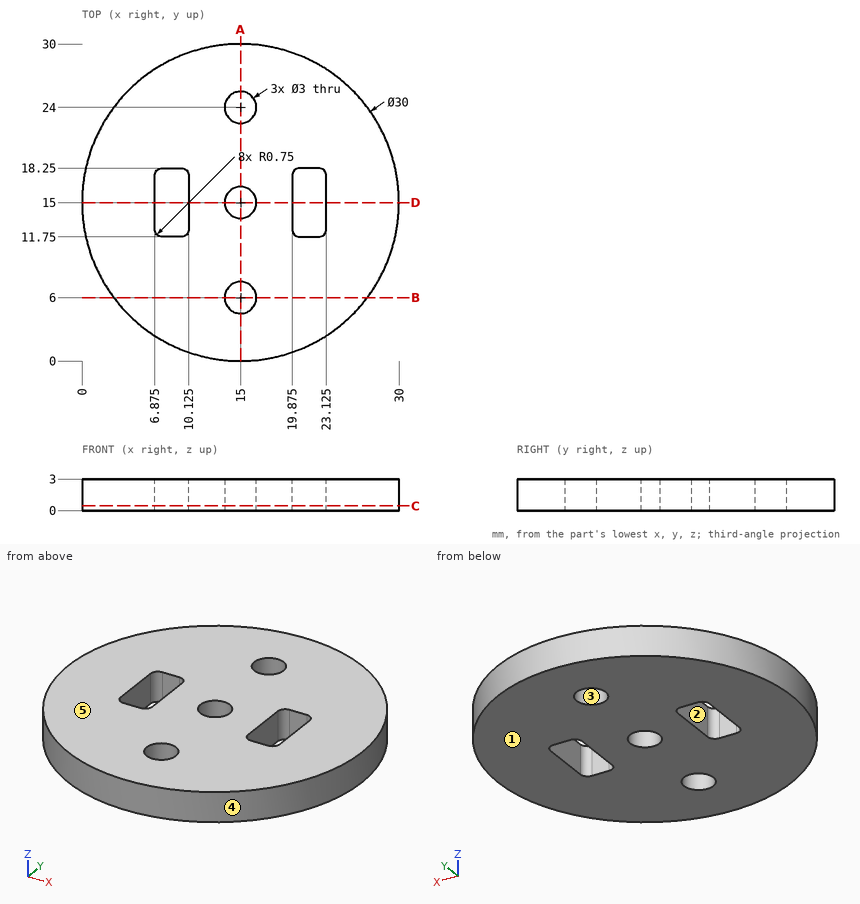
Geometry check sheet. Reference: drawing and pictorial views, mm from the part's lowest x, y, z. A direction names the side the tool comes from. Coordinates: 2 decimals unless noted, no trailing zeros. Order: outer loops, then holes, each group sorted by start corner. A loop starts at its lowest first (then second) coordinate and runs counter-clockwise, first axis right, second up. Notation, with made-up numbers: (54.25, -1.75) - (96.25, -1.75) arc R16 ccw to (96.25, 7.25) - close; hole circle Ø9 at (28.5, -37). An arc over 180 degrees is marked (long way). Answer in a Markdown table with one row per item. Add a question column.
1) Cross-section at A-A, the plane x = 15. Record the cut outline in (y, z), then the cut area to 3 significant figures.
2) Material ranges on line 1 along Y through (x, z) = (15, 2.1); line 2 along X through (y, z) = (17.75, 1.35); line 3 along Y through (x, z) = (8.25, 1.5), recorded low to high. Write a range as [from, to].
3) Set-up check for the marked faces 1 and 2: record each of +Z, -Z, +X, -X, +Y, -Y from which the full face is reachable in a straight line by a thin tool's end or side.
4) Cross-section at C-C, the plane z = 0.45. Record the cut outline in (x, y) (3 decimals).
5) Release check for a two-part mould opening along X. For the marked faces 3, 4 and 5 record: +X half, -X half, draft (parallel to the pull), parting line (faces both ways), or undercut.
6) Gauge pin test, flat ends, axial feed: P1, Ø2.5, axis at x = 15, y = 15, coming from the +Z side; P2, Ø0.9, axis at x = 8, z = 1, coming from the +Y side; P3, Ø1, axis at y = 23.5, z = 1.5, coming from the +X side; P4, Ø0.9, axis at y = 16, z = 1, coming from the +X side. Record the tip position at first contact, or that the pin passes through.
7) Cross-section at D-D, the plane y = 15. Record the cut outline in (x, z) (3 decimals), then the cut area to 3 significant figures.
8) Cross-section at B-B, the plane y = 6. Record the cut outline in (x, z), then the cut area to 3 significant figures.
Check result:
| question | item | result |
|---|---|---|
| 1 | outline | (0, 0) - (4.5, 0) - (4.5, 3) - (0, 3) - close; (7.5, 0) - (13.5, 0) - (13.5, 3) - (7.5, 3) - close; (16.5, 0) - (22.5, 0) - (22.5, 3) - (16.5, 3) - close; (25.5, 0) - (30, 0) - (30, 3) - (25.5, 3) - close |
| 1 | area | 63.0 mm² |
| 2 | line 1 | y = [0, 4.5], [7.5, 13.5], [16.5, 22.5], [25.5, 30] |
| 2 | line 2 | x = [0.25, 6.92], [10.08, 19.92], [23.08, 29.75] |
| 2 | line 3 | y = [1.6, 11.75], [18.25, 28.4] |
| 3 | face 1 | -Z, +X, -X, +Y, -Y |
| 3 | face 2 | +Z, -Z |
| 4 | outline | circle Ø30 at (15, 15); hole (6.875, 12.5) arc R0.75 ccw to (7.625, 11.75) - (9.375, 11.75) arc R0.75 ccw to (10.125, 12.5) - (10.125, 17.5) arc R0.75 ccw to (9.375, 18.25) - (7.625, 18.25) arc R0.75 ccw to (6.875, 17.5) - close; hole circle Ø3 at (15, 6); hole circle Ø3 at (15, 15); hole circle Ø3 at (15, 24); hole (19.875, 12.5) arc R0.75 ccw to (20.625, 11.75) - (22.375, 11.75) arc R0.75 ccw to (23.125, 12.5) - (23.125, 17.5) arc R0.75 ccw to (22.375, 18.25) - (20.625, 18.25) arc R0.75 ccw to (19.875, 17.5) - close |
| 5 | face 3 | undercut |
| 5 | face 4 | parting line |
| 5 | face 5 | draft |
| 6 | P1 | passes through |
| 6 | P2 | stops at y = 28.49 |
| 6 | P3 | stops at x = 27.69 |
| 6 | P4 | stops at x = 29.99 |
| 7 | outline | (0, 0) - (6.875, 0) - (6.875, 3) - (0, 3) - close; (10.125, 0) - (13.5, 0) - (13.5, 3) - (10.125, 3) - close; (16.5, 0) - (19.875, 0) - (19.875, 3) - (16.5, 3) - close; (23.125, 0) - (30, 0) - (30, 3) - (23.125, 3) - close |
| 7 | area | 61.5 mm² |
| 8 | outline | (3, 0) - (13.5, 0) - (13.5, 3) - (3, 3) - close; (16.5, 0) - (27, 0) - (27, 3) - (16.5, 3) - close |
| 8 | area | 63.0 mm² |
